from build123d import *

# Parameters (mm, degrees)
F1_DEPTH = 50


with BuildPart() as f1:
    # F0 (on Front) → F1 (new body)
    with BuildSketch(Plane.XZ):
        with BuildLine():
            Line((0, 0), (-75, 0))
            Line((-75, 0), (-75, -3.5))
            ThreePointArc((-75, -3.5), (-73.681981, -6.681981), (-70.5, -8))
            Line((-70.5, -8), (-17, -8))
            ThreePointArc((-17, -8), (-10.636039, -10.636039), (-8, -17))
            Line((-8, -17), (-8, -70.5))
            ThreePointArc((-8, -70.5), (-6.681981, -73.681981), (-3.5, -75))
            Line((-3.5, -75), (0, -75))
            Line((0, -75), (0, -50))
            Line((0, -50), (0, 0))
        make_face()
        with BuildLine():
            Line((2.5, -50), (0, -50))
            Line((0, -50), (0, -75))
            Line((0, -75), (0, -100))
            Line((0, -100), (50, -100))
            Line((50, -100), (50, -97.5))
            ThreePointArc((50, -97.5), (48.974874, -95.025126), (46.5, -94))
            Line((46.5, -94), (13, -94))
            ThreePointArc((13, -94), (8.050253, -91.949747), (6, -87))
            Line((6, -87), (6, -53.5))
            ThreePointArc((6, -53.5), (4.974874, -51.025126), (2.5, -50))
        make_face()
    extrude(amount=F1_DEPTH)


solid = f1.part
Verification items for the finished model (mm, model axes). A direction names the side the tool comes from. Round coordinates to 2 decimals unless told otherwise and drop trailing zeros. Order: outer loops, then holes, each group sorted by start corner. A loop starts at its lowest first (then second) coordinate and runs counter-clockwise, first axis right, second up.
1. Go/stop test with flat-tipped pins: P1, Ø15, axis at y = -13.5, z = -32, coming from the -X side; P2, Ø4, axis at y = -31, z = -12.5, coming from the -X side; P3, Ø15, axis at x = -56, y = -14, coming from the -Z side. Record where each tip stops, or that it passes through.
Final values:
P1: stops at x = -8
P2: stops at x = -10.78
P3: stops at z = -8
2. Access from +Z, -Z, +X, -X, +Y, -Y to the whole of each face (thin tool, end or side, straight path). Record for faces 4 (the flat face through (0, -25, -25)), 5 (the flat face through (-44, -25, -8)), 6 (the flat face through (-4, 0, -46)).
Final values:
face 4: +Z, +X, +Y, -Y
face 5: -Z, -X, +Y, -Y
face 6: +Z, -Z, +X, -X, +Y
3. Release check for a two-part mould opening along Z. For faces 1 (the flat face through (6, -25, -70)), 2 (the cylindrical face through (49, -24.65, -95.05)), 3 (the flat face through (-2, -25, -75)) record: +Z half, -Z half, draft (parallel to the pull), parting line (faces both ways), or undercut.
Final values:
face 1: draft
face 2: +Z half
face 3: -Z half
4. Section check C-C on x = -26. Record the cut outline in (y, z), then the cut area to 3 significant figures.
Final values:
outline: (-50, -8) - (0, -8) - (0, 0) - (-50, 0) - close
area: 400 mm2
5. Section check A-A on y = -37.5. Record the cut outline in (x, z), then the cut area to 3 significant figures.
Final values:
outline: (-75, -3.5) arc R4.5 ccw to (-70.5, -8) - (-17, -8) arc R9 cw to (-8, -17) - (-8, -70.5) arc R4.5 ccw to (-3.5, -75) - (0, -75) - (0, -100) - (50, -100) - (50, -97.5) arc R3.5 ccw to (46.5, -94) - (13, -94) arc R7 cw to (6, -87) - (6, -53.5) arc R3.5 ccw to (2.5, -50) - (0, -50) - (0, 0) - (-75, 0) - close
area: 1,710 mm2
6. Section check B-B on z = -27. Record the cut outline in (x, y).
Final values:
outline: (-8, -50) - (0, -50) - (0, 0) - (-8, 0) - close
7. Thickness scan on L1, parallel to Z at x = 20, y = -43; L2, parallel to Z at x = -28.5, y = -9. Record the ranges inside material, lowest first.
Final values:
L1: z = -100 to -94
L2: z = -8 to 0
